Answer from the drawing. Dimensions are ordinates in mm from the lowest x, y and z of the part. Round coordinates to 2 decimals unless told otherwise and drop trailing zeros. Write each loop counter-clockwise with the first axis right and the second up, starting at its lowest first coordinate (ties: lowest second). Pieces come first, ordered by that corner, then holes. Notation, with made-up numbers: (5.5, 48.25) - (63.5, 48.25) arc R18 cw to (63.5, 62.25) - close; hole circle Ø6 at (73.5, 67). An arc over 180 degrees is marked (long way). Write item = value, one per line. Start each with the question number.
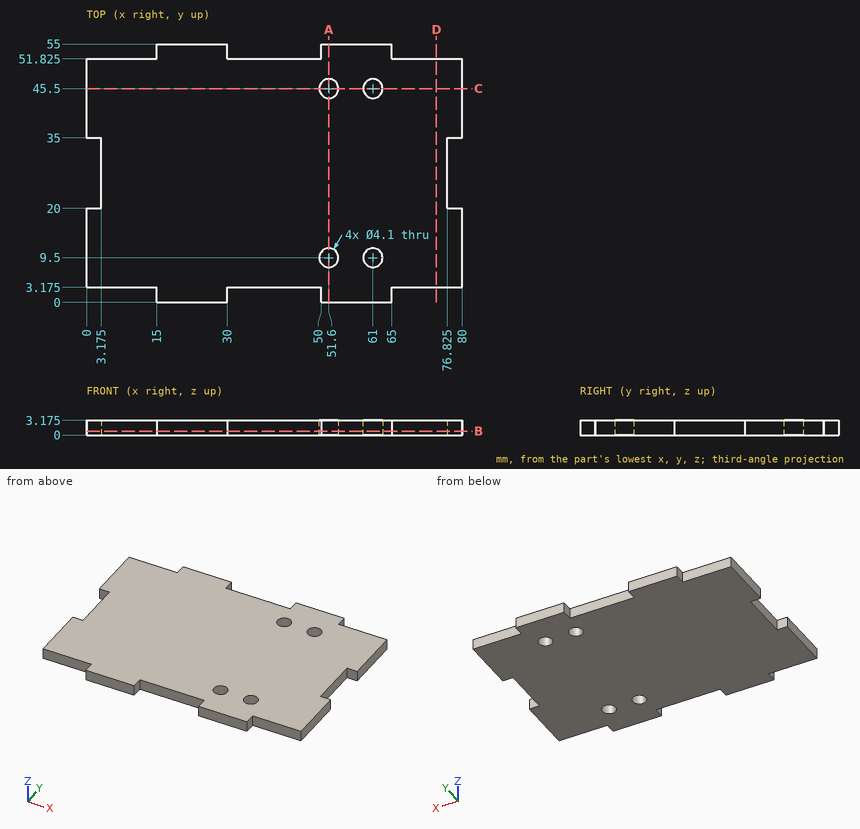
1. Find section C-C on y = 45.5. Give the vertices of the cut face in (x, z) (3 decimals).
2. Consider line 1 (Y direction, x = 61, z = 2.25); line 2 (Y direction, x = 53, z = 1.6); line 3 (Y direction, x = 68.5, z = 1.2) (3 decimals). Determine where each line is inside the solid, lowest interval first.
3. Each of these flat-tipped pins is pushed along its axis until it touches: pin 1 (12 mm diameter, centred on x = 25, y = 6, fed in from -Z); pin 2 (1.6 mm diameter, centred on x = 11, z = 1.5, fed in from -Y) (3 decimals); pin 3 (1.6 mm diameter, centred on y = 2, z = 1, fed in from +X); pin 4 (1 mm diameter, centred on x = 10, z = 2, fed in from +Y) (3 decimals). Where does it stop, or does it pass through?
4. Find section A-A on x = 51.6. Give the vertices of the cut face in (y, z) (3 decimals).
5. Find section B-B on z = 0.85. Give the number of separate pieces and of enclosed holes in the cut face, plus the area to 3 significant figures.
6. Find section D-D on x = 74.5. Give the vertices of the cut face in (y, z) (3 decimals), plus the area to 3 significant figures.
Answer key:
q1.outline = (0, 0) - (49.55, 0) - (49.55, 3.175) - (0, 3.175) - close; (53.65, 0) - (58.95, 0) - (58.95, 3.175) - (53.65, 3.175) - close; (63.05, 0) - (80, 0) - (80, 3.175) - (63.05, 3.175) - close
q2.line_1 = 0 to 7.45, 11.55 to 43.45, 47.55 to 55
q2.line_2 = 0 to 8, 11 to 44, 47 to 55
q2.line_3 = 3.175 to 51.825
q3.pin_1 = 0
q3.pin_2 = 3.175
q3.pin_3 = 65
q3.pin_4 = 51.825
q4.outline = (0, 0) - (7.45, 0) - (7.45, 3.175) - (0, 3.175) - close; (11.55, 0) - (43.45, 0) - (43.45, 3.175) - (11.55, 3.175) - close; (47.55, 0) - (55, 0) - (55, 3.175) - (47.55, 3.175) - close
q5.separate_pieces = 1
q5.enclosed_holes = 4
q5.area = 3,930 mm²
q6.outline = (3.175, 0) - (51.825, 0) - (51.825, 3.175) - (3.175, 3.175) - close
q6.area = 154 mm²
